Source: CAD feature listing. Evaluate the final solid. Frame: model axes, mm. A direction names the side the tool comes from. Give positions to 0.01 mm unless a question says otherwise; leave off trailing zeros. Order: outer loops, then holes, each group sorted by start corner. A loop starts at its lowest first (then second) coordinate and runs counter-clockwise, first axis right, second up.
from build123d import *

# Parameters (mm, degrees)
SKETCH2_R          = 3
CUT_EXTRUDE3_DEPTH = 12.5
CIRPATTERN1_COUNT  = 8


with BuildPart() as part:
    # Sketch1 → Revolve1 (revolve)
    with BuildSketch(Plane(origin=(0, 0, 0), x_dir=(0, 0, -1), z_dir=(1, 0, 0)), mode=Mode.PRIVATE) as revolve1_sk:
        with BuildLine():
            Line((0, 0), (0, -10))
            Line((0, -10), (18, -10))
            ThreePointArc((18, -10), (20, -8), (22, -10))
            Line((22, -10), (24, -10))
            ThreePointArc((24, -10), (26, -8), (28, -10))
            Line((28, -10), (35, -10))
            Line((35, -10), (35, 25))
            Line((35, 25), (15, 25))
            Line((15, 25), (15, 0))
            Line((15, 0), (0, 0))
        make_face()
    revolve(revolve1_sk.sketch.rotate(Axis((0, 25, -35), (0, 0, 1)), 180), axis=Axis((0, 25, -35), (0, 0, 1)))

    # Sketch2 → Cut-Extrude3 (cut, symmetric)
    with BuildSketch(Plane(origin=(0, 0, 0), x_dir=(1, 0, 0), z_dir=(0, 1, 0))):
        with Locations(Location((0, 8, 0), (0, 0, 270))):
            Circle(SKETCH2_R)
    cut_extrude3 = extrude(amount=CUT_EXTRUDE3_DEPTH, both=True, mode=Mode.SUBTRACT)

    # CirPattern1: Cut-Extrude3 ×8 about axis
    cirpattern1_axis = Axis((0, 25, -35), (0, 0, -1))
    for i in range(1, CIRPATTERN1_COUNT):
        add(cut_extrude3.rotate(cirpattern1_axis, i * 360 / CIRPATTERN1_COUNT), mode=Mode.SUBTRACT)


solid = part.part
1) Reachability of faces 5 (the face through (-23, 6, -7)), 6 (the face through (9.58, 48.09, -7.4)) from +Z, -Z, +X, -X, +Y, -Y: full face, straight path, thin tool, end or side. Return the list, or none.
Checks:
face 5: none
face 6: +Z
2) First-contact query: pin 1 Ø1.5 at (x, z) = (21, -15) entering from -Y; pin 2 Ø4 at (x, z) = (28, -29) entering from +Y; pin 3 Ø6 at (x, z) = (-16.5, -16.5) entering from +Y. Flat tips, straight axial feed; report the tip coordinate or a pass-through.
Checks:
pin 1: stops at y = -3.55
pin 2: stops at y = 48.43
pin 3: stops at y = 57.29
3) Ray query, L1, parallel to Z at x = 0, y = -4.25; L2, parallel to Z at x = -19, y = 11.5; L3, parallel to Y at x = -28.5, z = -7.5. Return the intervals inside material, ascending.
Checks:
L1: z = -35 to -11, -5 to 0
L2: z = -35 to -15
L3: y = 4.68 to 22.04, 27.96 to 45.32
4) Section query A-A on x = 0. Output: boundary loops of the cut face in (y, z).
Checks:
outline: (-10, -35) - (60, -35) - (60, -28) arc R2 cw to (60, -24) - (60, -22) arc R2 cw to (60, -18) - (60, -11) - (50, -11) - (50, -15) - (0, -15) - (0, -11) - (-10, -11) - (-10, -18) arc R2 cw to (-10, -22) - (-10, -24) arc R2 cw to (-10, -28) - close; (-10, -5) - (0, -5) - (0, 0) - (-10, 0) - close; (50, -5) - (60, -5) - (60, 0) - (50, 0) - close
5) Pull-direction query (Z, two-part tool) for faces 1 (the face through (20.285, 3.09, -5.229)), 2 (the face through (0, 25, -15)), 3 (the face through (0, 25, -35)), 4 (the face through (34.168, 17.413, -31.549)); classes: +Z half, -Z half, draft (parallel to the pull), parting line (faces both ways), or undercut.
Checks:
face 1: undercut
face 2: +Z half
face 3: -Z half
face 4: draft
6) Section query C-C on z = -2.5. Output: boundary loops of the cut face in (x, y), and give its area (3 significant figures).
Checks:
outline: circle Ø70 at (0, 25); hole circle Ø50 at (0, 25)
area: 1,880 mm2
7) Section query B-B on z = -8. State how many separate pieces and enclosed holes the cut face has, and give its area (3 significant figures).
Checks:
separate pieces: 8
enclosed holes: 0
area: 1,400 mm2
8) Section query D-D on z = -31. Output: boundary loops of the cut face in (x, y).
Checks:
outline: circle Ø70 at (0, 25)
